from build123d import *

# Parameters (mm, degrees)
ESQUISSE1_W                  = 10
ESQUISSE1_H                  = 10
BOSS_EXTRU_1_DEPTH           = 307
ENL_V_MAT_EXTRU_1_DEPTH      = 308.081422427
ENL_V_MAT_EXTRU_1_DEPTH_BACK = 308.081422427
ESQUISSE2_W                  = 10
ESQUISSE2_H                  = 22
D_GAGEMENT_M41_OUTLINE_W     = 10
D_GAGEMENT_M41_OUTLINE_H     = 10
D_GAGEMENT_M41_OUTLINE_R     = 2.15
D_GAGEMENT_M41_DEPTH         = 5
D_GAGEMENT_START             = -5
D_GAGEMENT_M41_2_OUTLINE_R   = 2.15
D_GAGEMENT_M41_2_DEPTH       = 5


# Read off the part's stored shape, not the designer's step: Dégagement M41
with BuildPart() as part:
    # Esquisse1 → Boss.-Extru.1 (new body)
    with BuildSketch(Plane.XY):
        Rectangle(ESQUISSE1_W, ESQUISSE1_H)
    extrude(amount=BOSS_EXTRU_1_DEPTH)

    # Esquisse2 → Enlèv. mat.-Extru.1 (cut, two sides: drawn at the far end of the back side and taken through both)
    with BuildSketch(Plane(origin=(0, 0, 0), x_dir=(1, 0, 0), z_dir=(0, 1, 0)).offset(-ENL_V_MAT_EXTRU_1_DEPTH_BACK)):
        with Locations((0, -11)):
            Rectangle(ESQUISSE2_W, ESQUISSE2_H)
    extrude(amount=ENL_V_MAT_EXTRU_1_DEPTH + ENL_V_MAT_EXTRU_1_DEPTH_BACK, mode=Mode.SUBTRACT)

    # Dégagement M41 outline → Dégagement M41 (cut)
    with BuildSketch(Plane.YZ):
        with Locations((0, 135)):
            Rectangle(D_GAGEMENT_M41_OUTLINE_W, D_GAGEMENT_M41_OUTLINE_H)
        with Locations((0, 31.09)):
            Circle(D_GAGEMENT_M41_OUTLINE_R)
        with Locations((0, 74.69)):
            Circle(D_GAGEMENT_M41_OUTLINE_R)
    extrude(amount=D_GAGEMENT_M41_DEPTH, mode=Mode.SUBTRACT)

    # D_gagement M41 2 outline → D_gagement M41 2 (cut)
    with BuildSketch(Plane.YZ.offset(D_GAGEMENT_START)):
        with Locations((0, 31.09)):
            Circle(D_GAGEMENT_M41_2_OUTLINE_R)
        with Locations((0, 74.69)):
            Circle(D_GAGEMENT_M41_2_OUTLINE_R)
    extrude(amount=D_GAGEMENT_M41_2_DEPTH, mode=Mode.SUBTRACT)


solid = part.part
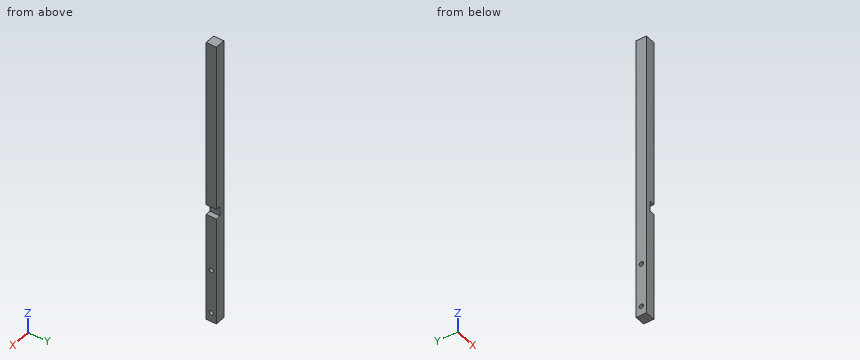
Source: CAD feature listing. Evaluate the final solid. Frame: model axes, mm. Give positions to 0.01 mm unless a question says otherwise; leave off trailing zeros. Write each loop counter-clockwise with the first axis right and the second up, starting at its lowest first coordinate (ties: lowest second). Pieces come first, ordered by that corner, then holes. Notation, with made-up numbers: M -7.5,38.25 L 0.5,38.25 A32 ccw 0.5,67.25 Z; hole C -33.5,-10.75 d9. An arc over 180 degrees is marked long. Return JSON: item names as keys, results as strings. Group by question number.
1) Ray query, L1, parallel to Z at x = 2.25, y = 0; L2, parallel to Z at x = -2.75, y = 0; L3, parallel to Z at x = 3.5, y = -4.25. Return the intervals inside material, ascending.
2) Cut plane B-B, the plane z = 135. Output: boundary loops of the cut face in (x, y), then the cut area to 3 significant figures.
3) Cut plane A-A, the plane y = 0. Output: boundary loops of the cut face in (x, z).
4) First-contact query: pin 1 Ø5 at (y, z) = (0, 134.5) entering from +X; pin 2 Ø3.5 at (y, z) = (0, 31.09) entering from -X. Flat tips, straight axial feed; report the tip coordinate or a pass-through.
Data:
{
 "1": {"L1": "z = 22 to 28.94, 33.24 to 72.54, 76.84 to 130, 140 to 307", "L2": "z = 22 to 28.94, 33.24 to 72.54, 76.84 to 307", "L3": "z = 22 to 130, 140 to 307"},
 "2": {"outline": "M -5,-5 L 0,-5 L 0,5 L -5,5 Z", "area": "50.0 mm²"},
 "3": {"outline": "M -5,22 L 5,22 L 5,28.94 L -5,28.94 Z; M -5,33.24 L 5,33.24 L 5,72.54 L -5,72.54 Z; M -5,76.84 L 5,76.84 L 5,130 L 0,130 L 0,140 L 5,140 L 5,307 L -5,307 Z"},
 "4": {"pin 1": "stops at x = 0", "pin 2": "passes through"}
}
